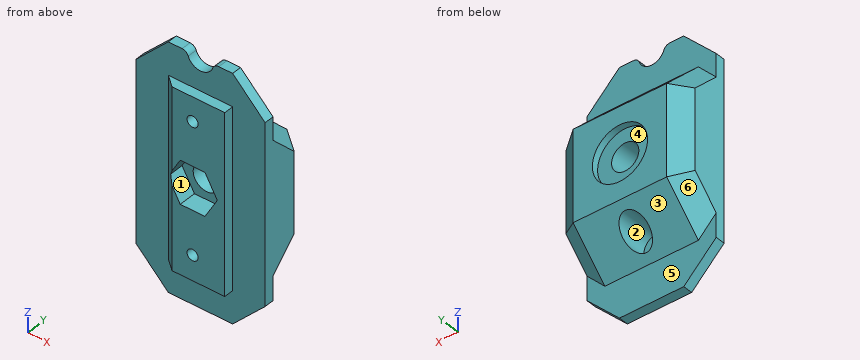
```python
from build123d import *
from OCP.BRepFilletAPI import BRepFilletAPI_MakeChamfer

# Parameters (mm, degrees)
SKETCH1_W           = 12.900022784
SKETCH1_H           = 55.1
SKETCH1_R           = 1.7
SKETCH1_W_2         = 6.899977216
BOSS_EXTRUDE1_DEPTH = 6
SKETCH2_R           = 2.1
BOSS_EXTRUDE2_DEPTH = 3
CHAMFER2_SIZE2      = 3
CHAMFER2_SIZE       = 3.575260778
SKETCH3_W           = 39.8
SKETCH3_H           = 24
BOSS_EXTRUDE3_DEPTH = 12
SKETCH5_R           = 4.2
CUT_EXTRUDE2_DEPTH  = 34
SKETCH7_R           = 4
CUT_EXTRUDE4_DEPTH  = 2
SKETCH10_R          = 4
CUT_EXTRUDE5_DEPTH  = 6
FILLET2_R           = 2
CUT_EXTRUDE6_DEPTH  = 5.4
CHAMFER3_SIZE       = 14
CHAMFER4_SIZE       = 4
CHAMFER4_SIZE2      = 5.505527682
SKETCH12_R          = 8.5
CUT_EXTRUDE7_DEPTH  = 2


# Some blends are built 0.0001 mm under size
with BuildPart() as part:
    # Sketch1 → Boss-Extrude1 (new body)
    # profile 1 of 2: a face of its own
    with BuildSketch(Plane.XZ.offset(561.298939869)):
        with Locations((-177.760855006, 568.270141885)):
            Rectangle(SKETCH1_W, SKETCH1_H)
        with Locations((-181.210843614, 548.420141885)):
            Circle(SKETCH1_R, mode=Mode.SUBTRACT)
        with Locations((-181.210843614, 588.420141885)):
            Circle(SKETCH1_R, mode=Mode.SUBTRACT)
    # profile 2 of 2: a face of its own
    with BuildSketch(Plane.XZ.offset(561.298939869)):
        with Locations((-187.660855006, 568.270141885)):
            Rectangle(SKETCH1_W_2, SKETCH1_H)
    extrude(amount=BOSS_EXTRUDE1_DEPTH)

    # Sketch2 → Boss-Extrude2 (add)
    with BuildSketch(Plane(origin=(0, -564.298939869, 0), x_dir=(1, 0, 0), z_dir=(0, 1, 0))):
        Polygon((-191.110843614, -530.720141885), (-171.310843614, -530.720141885), (-161.310843614, -540.720141885), (-161.310843614, -595.820141885), (-171.310843614, -605.820141885), (-191.110843614, -605.820141885), (-201.110843614, -595.820141885), (-201.110843614, -540.720141885), align=None)
        with Locations((-181.210843614, -548.420141885)):
            Circle(SKETCH2_R, mode=Mode.SUBTRACT)
        with Locations((-181.210843614, -588.420141885)):
            Circle(SKETCH2_R, mode=Mode.SUBTRACT)
    extrude(amount=BOSS_EXTRUDE2_DEPTH)

    # Chamfer2
    chamfer2_edges = [part.edges().sort_by_distance(p)[0] for p in [
        (-191.110843614, -567.298939869, 568.270141885),
    ]]
    chamfer2_side = [part.faces().sort_by_distance(p)[0] for p in [
        (-191.050843614, -567.298939869, 568.270141885),
    ]]
    chamfer(chamfer2_edges, length=CHAMFER2_SIZE - 0.0001, length2=CHAMFER2_SIZE2 - 0.0001, reference=chamfer2_side[0])  # a hair under: the kernel refuses the full size

    # Sketch3 → Boss-Extrude3 (add)
    with BuildSketch(Plane(origin=(0, -561.298939869, 0), x_dir=(1, 0, 0), z_dir=(0, 1, 0))):
        with Locations((-181.210843614, -568.420141885)):
            Rectangle(SKETCH3_W, SKETCH3_H)
    extrude(amount=BOSS_EXTRUDE3_DEPTH)

    # Sketch5 → Cut-Extrude2 (cut)
    with BuildSketch(Plane(origin=(0, -549.298939869, 0), x_dir=(1, 0, 0), z_dir=(0, 1, 0))):
        with Locations(Location((-181.210843614, -568.420141885, 0), (0, 0, 180))):
            Circle(SKETCH5_R)
    extrude(amount=-CUT_EXTRUDE2_DEPTH, mode=Mode.SUBTRACT)

    # Sketch7 → Cut-Extrude4 (cut)
    with BuildSketch(Plane(origin=(0, -561.298939869, 0), x_dir=(1, 0, 0), z_dir=(0, 1, 0))):
        with Locations(Location((-181.210843614, -548.420141885, 0), (0, 0, 180))):
            Circle(SKETCH7_R)
        with Locations(Location((-181.210843614, -588.420141885, 0), (0, 0, 180))):
            Circle(SKETCH7_R)
    extrude(amount=-CUT_EXTRUDE4_DEPTH, mode=Mode.SUBTRACT)

    # Sketch10 → Cut-Extrude5 (cut)
    with BuildSketch(Plane(origin=(0, -561.298939869, 0), x_dir=(1, 0, 0), z_dir=(0, 1, 0))):
        with Locations((-181.210843614, -605.820141885)):
            Circle(SKETCH10_R)
    extrude(amount=-CUT_EXTRUDE5_DEPTH, mode=Mode.SUBTRACT)

    # Fillet2
    fillet2_edges = [part.edges().sort_by_distance(p)[0] for p in [
        (-177.210843614, -562.798939869, 605.820141885),
        (-185.210843614, -562.798939869, 605.820141885),
    ]]
    fillet(fillet2_edges, radius=FILLET2_R)

    # Sketch11 → Cut-Extrude6 (cut)
    with BuildSketch(Plane.XZ.offset(567.298939869)):
        Polygon((-185.02135539, 575.020141885), (-188.831867167, 568.420141885), (-185.02135539, 561.820141885), (-177.400331837, 561.820141885), (-173.58982006, 568.420141885), (-177.400331837, 575.020141885), align=None)
    extrude(amount=-CUT_EXTRUDE6_DEPTH, mode=Mode.SUBTRACT)

    # Chamfer3
    # the kernel refuses this chamfer: 14 mm, written as the material it adds along each edge
    with BuildSketch(Plane(origin=(-161.310843614, -561.298939869, 580.420141885), x_dir=(0, -0.027495876610589963, 0.9996219169112966), z_dir=(-1, 0, 0))) as chamfer3_piece_1_section:
        Polygon((CHAMFER3_SIZE * 0.999621916911, CHAMFER3_SIZE * 0.0274958766106), (-CHAMFER3_SIZE * 0.0274958766106, CHAMFER3_SIZE * 0.999621916911), (0, 0), align=None)
    chamfer3_piece_1 = extrude(amount=39.8, mode=Mode.PRIVATE)
    chamfer3_piece_1 = chamfer3_piece_1 - Plane(origin=(-181.210843614, -559.739674618, 588.420141885), x_dir=(-1, 0, 0), z_dir=(0, 1, 0)) * Cylinder(4, 136, mode=Mode.PRIVATE)
    chamfer3_piece_1 = split(chamfer3_piece_1, bisect_by=Plane(origin=(-194.47751028, -549.298939869, 592.639373465), z_dir=(0, -1, 0)), keep=Keep.TOP, mode=Mode.PRIVATE)
    add(chamfer3_piece_1)
    with BuildSketch(Plane(origin=(-201.110843614, -561.298939869, 556.420141885), x_dir=(3.206917197373746e-15, 0.9996219169112968, 0.027495876610589966), z_dir=(1, 0, 0))) as chamfer3_piece_2_section:
        Polygon((CHAMFER3_SIZE * 0.999621916911, -CHAMFER3_SIZE * 0.0274958766106), (-CHAMFER3_SIZE * 0.0274958766106, -CHAMFER3_SIZE * 0.999621916911), (0, 0), align=None)
    chamfer3_piece_2 = extrude(amount=39.8, mode=Mode.PRIVATE)
    chamfer3_piece_2 = split(chamfer3_piece_2, bisect_by=Plane(origin=(-167.944176947, -549.298939869, 552.464896655), z_dir=(0, -1, 0)), keep=Keep.TOP, mode=Mode.PRIVATE)
    chamfer3_piece_2 = chamfer3_piece_2 - Plane(origin=(-181.210843614, -551.475687905, 548.420141885), x_dir=(-1, 0, 0), z_dir=(0, 1, 0)) * Cylinder(4, 136, mode=Mode.PRIVATE)
    add(chamfer3_piece_2)

    # Chamfer4: one chamfer whose edges measure the first distance from different faces: ONE call of the kernel's chamfer builder (chamfer() names one face for all edges)
    chamfer4_edges_1 = [part.edges().sort_by_distance(p)[0] for p in [
        (-161.310843614, -555.298939869, 588.420141885),
        (-161.310843614, -555.298939869, 548.420141885),
        (-161.310843614, -549.298939869, 568.420141885),
    ]]
    chamfer4_side_1 = [part.faces().sort_by_distance(p)[0] for p in [
        (-161.310843614, -557.666443356, 568.381717896),
    ]]
    chamfer4_edges_2 = [part.edges().sort_by_distance(p)[0] for p in [
        (-201.110843614, -555.298939869, 588.420141885),
        (-201.110843614, -555.298939869, 548.420141885),
        (-201.110843614, -549.298939869, 568.420141885),
    ]]
    chamfer4_side_2 = [part.faces().sort_by_distance(p)[0] for p in [
        (-201.110843614, -557.666443356, 568.381717896),
    ]]
    chamfer4 = BRepFilletAPI_MakeChamfer(part.part.solid().wrapped)
    for e in chamfer4_edges_1:
        chamfer4.Add(CHAMFER4_SIZE, CHAMFER4_SIZE2, e.wrapped, chamfer4_side_1[0].wrapped)  # the first distance lies on this face
    for e in chamfer4_edges_2:
        chamfer4.Add(CHAMFER4_SIZE, CHAMFER4_SIZE2, e.wrapped, chamfer4_side_2[0].wrapped)  # the first distance lies on this face
    add(Compound.cast(chamfer4.Shape()), mode=Mode.REPLACE)

    # Sketch12 → Cut-Extrude7 (cut)
    with BuildSketch(Plane(origin=(0, -549.298939869, 0), x_dir=(1, 0, 0), z_dir=(0, 1, 0))):
        with Locations(Location((-181.210843614, -568.420141885, 0), (0, 0, 180))):
            Circle(SKETCH12_R)
    extrude(amount=-CUT_EXTRUDE7_DEPTH, mode=Mode.SUBTRACT)


solid = part.part
```
Could you check a few things on this model? Use its own coordinates, in mm. Face numbers are marked on the shaded views. A direction names the side the tool comes from. Coordinates: 2 decimals unless noted, no trailing zeros. Order: outer loops, then holes, each group sorted by start corner. A loop starts at its lowest first (then second) coordinate and runs counter-clockwise, first axis right, second up. Notation, with made-up numbers: M 88,20.25 L 138,20.25 A24 cw 138,44.25 Z; hole C 34.5,-23.75 d3. An arc over 180 degrees is marked long. Use a Markdown table: item, result. Add a question column.
Q1. I want a section at B-B on y = -552.25. List the corners of the cut face in (x, z) for me.
Q2. Which directions (+Z, -Z, +X, -X, +Y, -Y) give clear straight access to the entire face, cutting with the end or side of a thin tool? Please do the marked faces 1, 2 and 3.
Q3. I want a section at D-D on y = -559.75. List the corners of the cut face in (x, z) for me, then the cut area to 3 significant figures.
Q4. I want a section at C-C on x = -194.5. List the corners of the cut face in (y, z) for me.
Q5. If I drill on L1, parallel to Y at x = -182, z = 591.5; L2, parallel to Y at x = -192, z = 557.5; L3, parallel to Z at x = -186, y = -565, over which ranges is the centre line in solid material (lowest first)?
Q6. We'd pull the mould along Z, two halves only. Please class the marked faces 4, 5 and 6: pulls with the +Z half, pulls with the -Z half, needs draft (parallel to the pull), parting line crosses it, or undercut.
Q7. I'm going to push flat-ended pins straight in: pin 1 (4 mm diameter, centred on x = -182.5, y = -553.5, fed in from -Z); pin 2 (4.5 mm diameter, centred on x = -181.5, y = -564.5, fed in from +Z); pin 3 (1.5 mm diameter, centred on y = -566, z = 575.5, fed in from +X). Where does each tip first touch, or does it pass through?
Checked values:
| question | item | result |
|---|---|---|
| 1 | outline | M -199.67,555.64 L -195.61,551.47 L -183.8,551.47 A4 cw -178.62,551.47 L -166.82,551.47 L -162.75,555.64 L -162.75,581.2 L -166.82,585.37 L -178.62,585.37 A4 cw -183.8,585.37 L -195.61,585.37 L -199.67,581.2 Z; hole C -181.21,568.42 d8.4 |
| 2 | face 1 | -Y |
| 2 | face 2 | +Y |
| 2 | face 3 | -Z, +X, -X, +Y |
| 3 | outline | M -201.11,549.63 L -195.61,543.97 L -166.82,543.97 L -161.31,549.63 L -161.31,587.21 L -166.82,592.87 L -195.61,592.87 L -201.11,587.21 Z; hole C -181.21,568.42 d8.4; hole C -181.21,548.42 d8; hole C -181.21,588.42 d8 |
| 3 | area | 1,730 mm² |
| 4 | outline | M -564.3,534.11 L -561.3,534.11 L -561.3,542.42 L -549.3,554.42 L -549.3,582.42 L -561.3,594.42 L -561.3,602.43 L -564.3,602.43 Z |
| 5 | L1 | -567.3 to -563.3 |
| 5 | L2 | -564.3 to -549.3 |
| 5 | L3 | 540.72 to 563.52, 573.33 to 595.82 |
| 6 | face 4 | undercut |
| 6 | face 5 | needs draft |
| 6 | face 6 | pulls with the -Z half |
| 7 | pin 1 | z = 550.7 |
| 7 | pin 2 | z = 602.72 |
| 7 | pin 3 | x = -171.31 |
